```python
from build123d import *

# Parameters (mm, degrees)
BOSS_EXTRUDE1_DEPTH = 179.605122421
CHAMFER2_SIZE       = 0.5
CHAMFER2_SIZE2      = 0.353553391
CHAMFER1_SIZE       = 0.5
CUT_EXTRUDE1_REACH  = 182.992


with BuildPart() as part:
    # Sketch1 → Boss-Extrude1 (new body)
    with BuildSketch(Plane.XY):
        with BuildLine():
            Line((5.5, 6.829360749), (2.570639251, 3.9))
            Line((2.570639251, 3.9), (0, 3.9))
            Line((0, 3.9), (0, 2.1))
            ThreePointArc((0, 2.1), (0.803635208, 1.940147018), (1.48492424, 1.48492424))
            Line((1.48492424, 1.48492424), (10, 10))
            Line((10, 10), (4.5, 10))
            Line((4.5, 10), (2.62, 8.12))
            Line((2.62, 8.12), (5.5, 8.12))
            Line((5.5, 8.12), (5.5, 6.829360749))
        make_face()
    extrude(amount=BOSS_EXTRUDE1_DEPTH)

    # Chamfer2
    chamfer2_edges = [part.edges().sort_by_distance(p)[0] for p in [
        (2.62, 8.12, 89.802561211),
    ]]
    chamfer2_side = [part.faces().sort_by_distance(p)[0] for p in [
        (3.56, 9.06, 89.802561211),
    ]]
    chamfer(chamfer2_edges, length=CHAMFER2_SIZE, length2=CHAMFER2_SIZE2, reference=chamfer2_side[0])

    # Mirror1: part across plane


with BuildPart() as part_1:
    add(part.part)
    add(part.part.mirror(Plane(origin=(10, 10, 179.605122421), x_dir=(0, 0, 1), z_dir=(-0.707106781186544, 0.7071067811865511, 0))))

    # Chamfer1
    chamfer1_edges = [part_1.edges().sort_by_distance(p)[0] for p in [
        (10, 10, 89.802561211),
    ]]
    chamfer(chamfer1_edges, length=CHAMFER1_SIZE)

    # Mirror4: part across plane


with BuildPart() as part_2:
    add(part_1.part)
    add(part_1.part.mirror(Plane(origin=(0, 3.9, 179.605122421), x_dir=(0, 0, 1), z_dir=(1, 0, 0))))

    # Mirror5: part across plane


with BuildPart() as part_3:
    add(part_2.part)
    add(part_2.part.mirror(Plane(origin=(-3.9, 0, 179.605122421), x_dir=(0, 0, 1), z_dir=(0, 1, 0))))

    # Cut-Extrude1: up to this face of the body (flat: up to its plane)
    cut_extrude1_end = Plane(part_3.part.faces().sort_by_distance((-10, 7, 89.802561211))[0])
    # Sketch2 → Cut-Extrude1 (cut, up to the picked face)
    with BuildSketch(Plane(origin=(10, 0, 0), x_dir=(0, 0, -1), z_dir=(1, 0, 0)), mode=Mode.PRIVATE) as cut_extrude1_sk1:
        Polygon((0, -10), (-20, 10), (0, 10), align=None)
    cut_extrude1_tool1 = split(extrude(cut_extrude1_sk1.sketch, amount=-CUT_EXTRUDE1_REACH, mode=Mode.PRIVATE), bisect_by=cut_extrude1_end, keep=Keep.BOTH, mode=Mode.PRIVATE)
    # Sketch2 → Cut-Extrude1 (cut, up to the picked face)
    with BuildSketch(Plane(origin=(10, 0, 0), x_dir=(0, 0, -1), z_dir=(1, 0, 0)), mode=Mode.PRIVATE) as cut_extrude1_sk2:
        Polygon((-159.605122421, 10), (-179.605122421, 10), (-179.605122421, -10), align=None)
    cut_extrude1_tool2 = split(extrude(cut_extrude1_sk2.sketch, amount=-CUT_EXTRUDE1_REACH, mode=Mode.PRIVATE), bisect_by=cut_extrude1_end, keep=Keep.BOTH, mode=Mode.PRIVATE)
    add(cut_extrude1_tool1.solids().sort_by(Axis((10, 3.333333, 6.666667), (-1, 0, 0)))[0], mode=Mode.SUBTRACT)
    add(cut_extrude1_tool2.solids().sort_by(Axis((10, 3.333333, 172.938456), (-1, 0, 0)))[0], mode=Mode.SUBTRACT)


solid = part_3.part
```
Input: part model. Units: mm. Frame: model coordinates. A direction names the side the tool comes from. Round coordinates to 2 decimals unless told otherwise and drop trailing zeros. Write each question's results on one line, items separated by ' | '.
1. First-contact query: P1, Ø0.8, axis at y = 4, z = 127.5, coming from the -X side; P2, Ø2.5, axis at x = -1, z = 51, coming from the -Y side; P3, Ø2, axis at x = 5, y = -7, coming from the +Z side; P4, Ø8, axis at y = -1, z = 22.5, coming from the +X side. Flat tips, straight axial feed; report the tip coordinate or a pass-through.
Geometry results:
P1: x = -9.9 | P2: y = -3.9 | P3: z = 177.47 | P4: x = 10
2. Set-up query: faces 1 (the face through (0, 3.9, 89)), 2 (the face through (-5.39, -4.06, 88.61)), 3 (the face through (0, -3.9, 89)), 4 (the face through (3.9, 0, 89)). Return all of +Z, -Z, +X, -X, +Y, -Y with unobstructed straight access to the full face (end or side cutting, diameter ignored); none if empty.
Geometry results:
face 1: +Z, -Z, +Y | face 2: +Z, -Z | face 3: +Z, -Z, -Y | face 4: +Z, -Z, +X
3. Mould query, pull axis Y, two halves, no side actions, for faces 5 (the face through (-4.06, 5.39, 88.74)), 6 (the face through (-7, -10, 89)), 7 (the face through (5.39, -4.06, 88.61)), 8 (the face through (2.362, -0.14, 169.745)). Classes: +Y half, -Y half, draft (parallel to the pull), parting line (faces both ways), or undercut.
Geometry results:
face 5: undercut | face 6: -Y half | face 7: undercut | face 8: +Y half
4. Ray query, line 1 (X direction, y = -3.75, z = 96.5); line 2 (Y direction, x = -0.25, z = 23); line 3 (Y direction, x = -4, z = 51). Return the intervals inside material, ascending. Write a range as from..to.
Geometry results:
line 1: -9.25..-8.12, -5.08..5.08, 8.12..9.25 | line 2: -3.9..-2.09, 2.09..3.9 | line 3: -9.5..-8.12, -5.33..-2.67, 2.67..5.33, 8.12..9.5
